```python
from build123d import *

# Parameters (mm, degrees)
SKETCH1_W           = 133.35
SKETCH1_H           = 31.25
BOSS_EXTRUDE1_DEPTH = 0.7
SKETCH2_R           = 0.75
CUT_EXTRUDE1_DEPTH  = 1.4
FILLET1_R           = 1.25
FILLET2_R           = 0.5


with BuildPart() as part:
    # Sketch1 → Boss-Extrude1 (new body, symmetric)
    with BuildSketch(Plane.XY):
        Rectangle(SKETCH1_W, SKETCH1_H)
    extrude(amount=BOSS_EXTRUDE1_DEPTH, both=True)

    # Sketch2 → Cut-Extrude1 (cut)
    with BuildSketch(Plane.XY.offset(0.7)):
        Polygon((66.675, -15.625), (66.675, -15.125), (40.375, -15.125), (30.175, -15.625), align=None)
        Polygon((-34.425, -15.125), (-66.675, -15.125), (-66.675, -15.625), (-24.225, -15.625), align=None)
        with BuildLine():
            Line((-65.225, 1.975), (-66.675, 1.975))
            Line((-66.675, 1.975), (-66.675, -1.025))
            Line((-66.675, -1.025), (-65.225, -1.025))
            ThreePointArc((-65.225, -1.025), (-64.694669914, -0.805330086), (-64.475, -0.275))
            Line((-64.475, -0.275), (-64.475, 1.225))
            ThreePointArc((-64.475, 1.225), (-64.694669914, 1.755330086), (-65.225, 1.975))
        make_face()
        with BuildLine():
            Line((-65.225, -4.625), (-66.675, -4.625))
            Line((-66.675, -4.625), (-66.675, -7.625))
            Line((-66.675, -7.625), (-65.225, -7.625))
            ThreePointArc((-65.225, -7.625), (-64.694669914, -7.405330086), (-64.475, -6.875))
            Line((-64.475, -6.875), (-64.475, -5.375))
            ThreePointArc((-64.475, -5.375), (-64.694669914, -4.844669914), (-65.225, -4.625))
        make_face()
        with BuildLine():
            Line((66.675, -1.025), (66.675, 1.975))
            Line((66.675, 1.975), (65.225, 1.975))
            ThreePointArc((65.225, 1.975), (64.694669914, 1.755330086), (64.475, 1.225))
            Line((64.475, 1.225), (64.475, -0.275))
            ThreePointArc((64.475, -0.275), (64.694669914, -0.805330086), (65.225, -1.025))
            Line((65.225, -1.025), (66.675, -1.025))
        make_face()
        with BuildLine():
            Line((66.675, -7.625), (66.675, -4.625))
            Line((66.675, -4.625), (65.225, -4.625))
            ThreePointArc((65.225, -4.625), (64.694669914, -4.844669914), (64.475, -5.375))
            Line((64.475, -5.375), (64.475, -6.875))
            ThreePointArc((64.475, -6.875), (64.694669914, -7.405330086), (65.225, -7.625))
            Line((65.225, -7.625), (66.675, -7.625))
        make_face()
        with BuildLine():
            Line((4.825, -15.625), (6.325, -15.625))
            Line((6.325, -15.625), (6.325, -12.525))
            ThreePointArc((6.325, -12.525), (5.575, -11.775), (4.825, -12.525))
            Line((4.825, -12.525), (4.825, -15.625))
        make_face()
        with Locations((-64.75, -12.825)):
            Circle(SKETCH2_R)
        with Locations((64.75, -12.825)):
            Circle(SKETCH2_R)
    extrude(amount=-CUT_EXTRUDE1_DEPTH, mode=Mode.SUBTRACT)

    # Fillet1
    fillet1_edges = [part.edges().sort_by_distance(p)[0] for p in [
        (-66.675, 15.625, 0),
        (66.675, 15.625, 0),
    ]]
    fillet(fillet1_edges, radius=FILLET1_R)

    # Fillet2
    fillet2_edges = [part.edges().sort_by_distance(p)[0] for p in [
        (6.325, -15.625, 0),
        (4.825, -15.625, 0),
        (40.375, -15.125, 0),
        (66.675, -15.125, 0),
        (30.175, -15.625, 0),
        (-34.425, -15.125, 0),
        (-24.225, -15.625, 0),
        (-66.675, -15.125, 0),
    ]]
    fillet(fillet2_edges, radius=FILLET2_R)


solid = part.part
```
Geometry check sheet. Reference: the model listing, model coordinates, mm. Round coordinates to 2 decimals unless told otherwise and drop trailing zeros. Loops run counter-clockwise (first coordinate to the right, second up) from the corner with the lowest first, then second, coordinate; pieces in that order, holes last. Notation, with made-up numbers: (39, 77) -> (70, 77) arc R26 cw to (70, 112) -> close; hole circle Ø1 at (-13, 70). An arc over 180 degrees is marked (long way). Use a Markdown table: item, result.
(1) Sectioned sample at A-A (x = -52). Enter the section's corners in (y, z) (3 decimals), then the cut area to 4 significant figures.
Calculated:
| item | result |
|---|---|
| outline | (-15.125, -0.7) -> (15.625, -0.7) -> (15.625, 0.7) -> (-15.125, 0.7) -> close |
| area | 43.05 mm² |
(2) Scan lines: probe 1 along Y at (x, z) = (-64.75, -0.4) (3 decimals); probe 2 along X at (y, z) = (-14, -0.4) (3 decimals); probe 3 along X at (y, z) = (14.5, 0.15). Record each from-to range of solid material in increasing order.
Calculated:
| item | result |
|---|---|
| probe 1 | -15.125 to -13.575, -12.075 to -7.455, -4.795 to -0.855, 1.805 to 15.625 |
| probe 2 | -66.675 to 4.825, 6.325 to 66.675 |
| probe 3 | -66.67 to 66.67 |
(3) Sectioned sample at B-B (z = 0.3). Give the number of separate pieces and of enclosed holes in the cut face, then the cut area to 3 significant figures.
Calculated:
| item | result |
|---|---|
| separate pieces | 1 |
| enclosed holes | 2 |
| area | 4,100 mm² |
(4) Go/stop test with flat-tipped pins: P1, Ø0.7, axis at x = 53, z = -0.5, coming from the -Y side (3 decimals); P2, Ø2, axis at x = 64.75, y = -12.825, coming from the +Z side; P3, Ø0.7, axis at y = 0.5, z = 0, coming from the -X side (3 decimals). Record where each tip stops, or that it passes through.
Calculated:
| item | result |
|---|---|
| P1 | y = -15.125 |
| P2 | z = 0.7 |
| P3 | x = -64.475 |
